Geometry check sheet. Reference: the model listing, model coordinates, mm. Face numbers are marked on the shaded views. A direction names the side the tool comes from. Coordinates: 2 decimals unless noted, no trailing zeros. Loops run counter-clockwise (first coordinate to the right, second up) from the corner with the lowest first, then second, coordinate; pieces in that order, holes last.
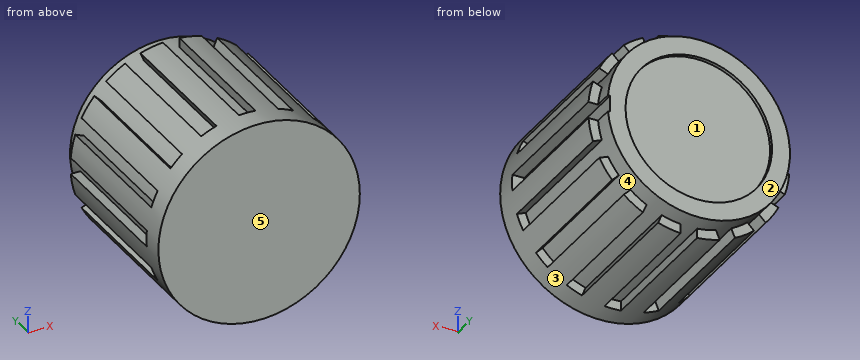
Autodesk Inventor part; units mm, degrees
ref_plane "YZ Plane" through (0, 0, 0) normal (1, 0, 0) x (0, 1, 0)
ref_plane "XZ Plane" through (0, 0, 0) normal (0, 1, 0) x (-1, 0, 0)
ref_plane "XY Plane" through (0, 0, 0) normal (0, 0, 1) x (1, 0, 0)
sketch "Sketch1" plane through (0, 0, 0) normal (0, 1, 0) x (-1, 0, 0)
  circle A0 centre (0, 0) radius 6.985
  dimension "d0" = 13.97
extrude "Extrusion1" add sketch "Sketch1" along normal blind 12.573
sketch "Sketch2" plane through (0, 12.573, 0) normal (0, 1, 0) x (1, 0, 0)
  circle A0 centre (0, 0) radius 6.3246
  circle A1 centre (0, 0) radius 6.985
  dimension "d3" = 12.6492
extrude "Extrusion2" cut sketch "Sketch2" against normal blind 1.27
sketch "Sketch3" plane through (0, 11.303, 0) normal (0, 1, 0) x (1, 0, 0)
  circle A0 centre (0, 0) radius 6.3246
  circle A1 centre (0, 0) radius 6.985
  circle A2 centre (0, 0) radius 6.985
  line L0 (-6.9616, -0.5715) -> (-6.2987, -0.5715)
  line L1 (-6.9616, 0.5715) -> (-6.2987, 0.5715)
  dimension "d6" = 1.143
  dimension "d7" = 0.5715
extrude "Extrusion3" cut sketch "Sketch3" against normal blind 9.779 contours A0 L0 A1 L1 picked at (-6.5273, 0.4446)
pattern_circular "Circular Pattern1" count 16 over 360 about axis through (0, 0, 0) along (0, 1, 0) of "Extrusion3"
sketch "Sketch4" plane through (0, 12.573, 0) normal (0, 1, 0) x (1, 0, 0)
  circle A0 centre (0, 0) radius 5.08
  dimension "d13" = 10.16
extrude "Extrusion4" cut sketch "Sketch4" against normal blind 0.254
sketch "Sketch5" plane through (0, 12.573, 0) normal (0, 1, 0) x (1, 0, 0)
  line L0 (6.2987, 0.5715) -> (6.9616, 0.5715)
  line L1 (6.9616, -0.5715) -> (6.2987, -0.5715)
  circle A0 centre (0, 0) radius 6.3246
  line L2 (6.2987, 0.5715) -> (6.1474, 0.5715)
  line L3 (6.1474, 0.5715) -> (6.1474, -0.5715)
  line L4 (6.1474, -0.5715) -> (6.2987, -0.5715)
extrude "Extrusion5" cut sketch "Sketch5" against normal blind 11.049 contours A0 L4 L3 L2 picked at (6.2065, 0)
properties part number "Knob3"
(1) Sectioned sample at C-C on y = 1. Record the cut outline in (x, z) (3 decimals), and give its area (3 significant figures).
Findings:
outline: circle Ø13.97 at (0, 0)
area: 153 mm2
(2) Gauge pin test, flat ends, axial feed: pin 1 Ø5 at (x, y) = (4, 2) entering from -Z; pin 2 Ø1 at (y, z) = (9.5, 0.5) entering from -X; pin 3 Ø6 at (y, z) = (10.5, -1.5) entering from +X. Record the tip position at first contact, or that the pin passes through.
Findings:
pin 1: stops at z = -6.82
pin 2: stops at x = -6.96
pin 3: stops at x = 6.96
(3) Sectioned sample at B-B on x = 0. Record the cut outline in (y, z) (3 decimals), and give its area (3 significant figures).
Findings:
outline: (0, -6.985) - (1.524, -6.985) - (1.524, -6.325) - (12.573, -6.325) - (12.573, -5.08) - (12.319, -5.08) - (12.319, 5.08) - (12.573, 5.08) - (12.573, 6.325) - (1.524, 6.325) - (1.524, 6.985) - (0, 6.985) - close
area: 158 mm2
(4) Sectioned sample at A-A on z = 0. Record the cut outline in (x, y) (3 decimals), and give its area (3 significant figures).
Findings:
outline: (-6.985, 0) - (6.985, 0) - (6.985, 1.524) - (6.147, 1.524) - (6.147, 12.573) - (5.08, 12.573) - (5.08, 12.319) - (-5.08, 12.319) - (-5.08, 12.573) - (-6.325, 12.573) - (-6.325, 1.524) - (-6.985, 1.524) - close
area: 157 mm2
(5) Scan lines: L1, parallel to Z at x = 0, y = 12.4; L2, parallel to X at y = 6.75, z = -4.25; L3, parallel to X at y = 12.45, z = 0. Record each from-to range of solid material in increasing order.
Findings:
L1: z = -6.32 to -5.08, 5.08 to 6.32
L2: x = -5.54 to -5.06, -4.68 to 4.68, 5.06 to 5.54
L3: x = -6.32 to -5.08, 5.08 to 6.15
(6) Access from +Z, -Z, +X, -X, +Y, -Y to the whole of each face (thin tool, end or side, straight path). Record for the marked faces 4 and 5.
Findings:
face 4: +Y
face 5: +Z, -Z, +X, -X, -Y
(7) Sectioned sample at D-D on z = -4.25. Record the cut outline in (x, y).
Findings:
outline: (-5.54, 0) - (5.54, 0) - (5.54, 11.3) - (5.06, 11.3) - (5.06, 1.52) - (4.68, 1.52) - (4.68, 12.57) - (2.78, 12.57) - (2.78, 12.32) - (-2.78, 12.32) - (-2.78, 12.57) - (-4.68, 12.57) - (-4.68, 1.52) - (-5.06, 1.52) - (-5.06, 11.3) - (-5.54, 11.3) - close
(8) Draft check along X on the marked faces 1, 2 and 3. Enter one of: +X half, -X half, draft (parallel to the pull), parting line (faces both ways), or undercut.
Findings:
face 1: undercut
face 2: draft
face 3: parting line
